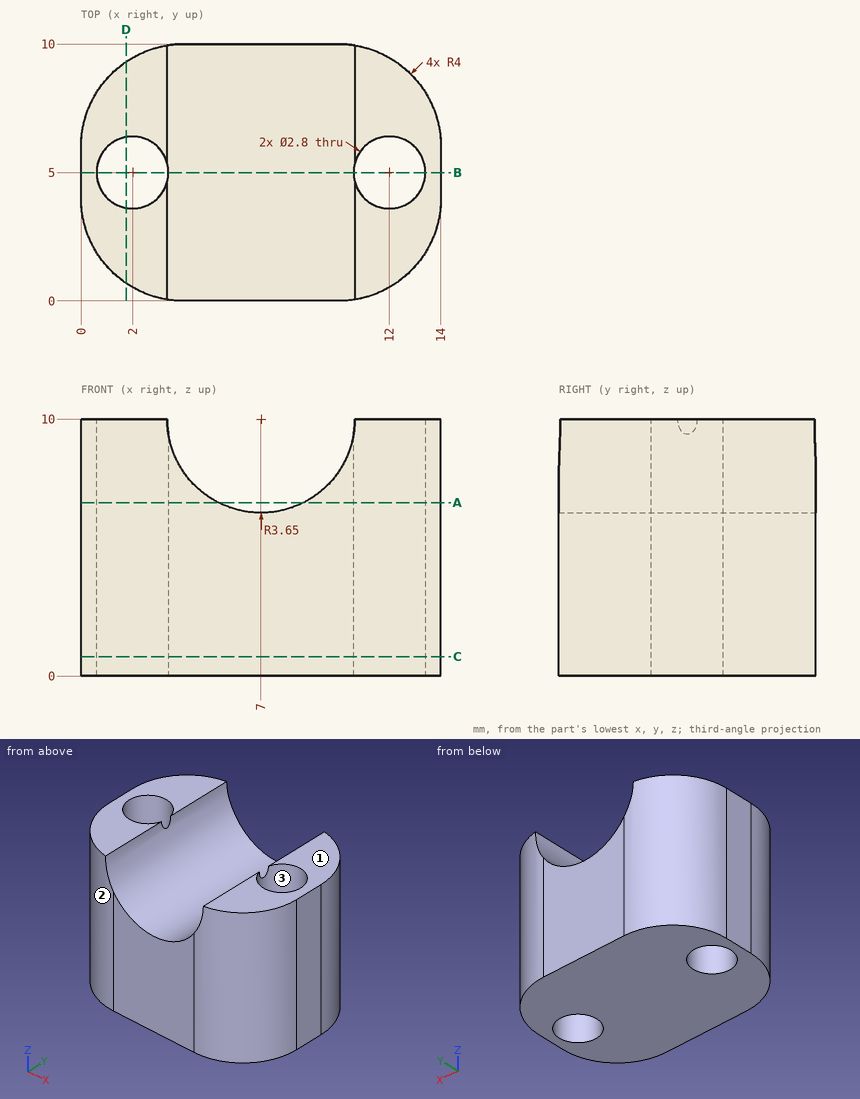
For this review, use the dimensioned drawing (mm, ordinates from the lowest corner) and the shaded views. Round coordinates to 2 decimals unless told otherwise and drop trailing zeros. Write each loop counter-clockwise with the first axis right and the second up, starting at its lowest first coordinate (ties: lowest second). Pieces come first, ordered by that corner, then holes. Notation, with made-up numbers: (55, 77) - (82, 77) arc R17 cw to (82, 86) - close; hole circle Ø10 at (-28.75, 42). An arc over 180 degrees is marked (long way). Answer as CSV lines item,"result". Start each with the question number.
(1) We need section C-C on z = 0.75. State the section outline as (x, y) points.
(2) We need section A-A on z = 6.75. State the section outline as (x, y) points.
(3) For pin 1 Ø4 at (x, y) = (8, 7.5) entering from +Z; pin 2 Ø1 at (y, z) = (1.5, 4.5) entering from +X; pin 3 Ø1 at (y, z) = (8, 4.5) entering from -X; pin 4 Ø1.7 at (x, y) = (2, 5) entering from +Z, all flat-tipped, find the tip position at first contact; note any pin that passes through.
(4) To check wall thickness, follow line 1 (X direction, y = 5.75, z = 7.75); line 2 (Y direction, x = 12, z = 3.25); line 3 (Y direction, x = 1.5, z = 2). State the ranges of each line that lie inside material, in increasing order.
(5) We need section B-B on y = 5. State the section outline as (x, z) points.
(6) We need section D-D on x = 1.75. State the section outline as (y, z) points, plus the area to 3 significant figures.
(7) Draft analysis for pull direction Y (two halves, no side actions). For the marked faces 1, 2 and 3, state which applies: pulls with the +Y half, pulls with the -Y half, needs draft (parallel to the pull), parting line crosses it, or undercut.
Worked answers:
1,outline,"(0, 4) arc R4 ccw to (4, 0) - (10, 0) arc R4 ccw to (14, 4) - (14, 6) arc R4 ccw to (10, 10) - (4, 10) arc R4 ccw to (0, 6) - close; hole circle Ø2.8 at (2, 5); hole circle Ø2.8 at (12, 5)"
2,outline,"(0, 4) arc R4 ccw to (4, 0) - (5.34, 0) - (5.34, 10) - (4, 10) arc R4 ccw to (0, 6) - close; (8.66, 0) - (10, 0) arc R4 ccw to (14, 4) - (14, 6) arc R4 ccw to (10, 10) - (8.66, 10) - close; hole circle Ø2.8 at (2, 5); hole circle Ø2.8 at (12, 5)"
3,pin 1,"z = 7.92"
3,pin 2,"x = 13.46"
3,pin 3,"x = 0.29"
3,pin 4,"through"
4,line 1,"0 to 0.82, 3.18 to 4.13, 9.87 to 10.82, 13.18 to 14"
4,line 2,"0.54 to 3.6, 6.4 to 9.46"
4,line 3,"0.88 to 3.69, 6.31 to 9.12"
5,outline,"(0, 0) - (0.6, 0) - (0.6, 10) - (0, 10) - close; (3.4, 0) - (10.6, 0) - (10.6, 9.4) arc R3.65 cw to (3.4, 9.4) - close; (13.4, 0) - (14, 0) - (14, 10) - (13.4, 10) - close"
6,outline,"(0.69, 0) - (3.62, 0) - (3.62, 10) - (0.69, 10) - close; (6.38, 0) - (9.31, 0) - (9.31, 10) - (6.38, 10) - close"
6,area,"58.6 mm²"
7,face 1,"needs draft"
7,face 2,"pulls with the -Y half"
7,face 3,"undercut"
